Work out the finished part from the listing and answer in its coordinate system (mm). A direction names the side the tool comes from. Give positions to 0.01 mm unless a question says otherwise; leave off trailing zeros. Order: outer loops, then holes, each group sorted by start corner. A loop starts at its lowest first (then second) coordinate and runs counter-clockwise, first axis right, second up. Notation, with made-up numbers: M 25,40 L 74,40 A31 cw 74,77 Z; hole C 84,-30 d11. An arc over 180 degrees is marked long. One line per item, written item: value.
Autodesk Inventor part; units mm, degrees
ref_plane "YZ Plane" through (0, 0, 0) normal (1, 0, 0) x (0, 1, 0)
ref_plane "XZ Plane" through (0, 0, 0) normal (0, 1, 0) x (-1, 0, 0)
ref_plane "XY Plane" through (0, 0, 0) normal (0, 0, 1) x (1, 0, 0)
sketch "Sketch1" plane through (0, 0, 0) normal (0, 1, 0) x (-1, 0, 0)
  line L0 (7.8, 0) -> (7.8, -7.8)
  line L1 (7.8, -7.8) -> (-7.8, -7.8)
  line L2 (-7.8, -7.8) -> (-7.8, 7.8)
  line L3 (-7.8, 7.8) -> (7.8, 7.8)
  line L4 (7.8, 7.8) -> (7.8, 0)
  line L5 (7.8, 7.8) -> (7, 7.8)
  line L6 (-7.8, 7.8) -> (-7.8, 7.4)
  line L7 (-7.8, -7.8) -> (-7.4, -7.8)
  line L8 (7.8, -7.8) -> (7.8, -7.4)
  line L9 (0, 0) -> (7.4, 0)
  line L10 (7.4, 0) -> (7.4, -7.4)
  line L11 (7.4, -7.4) -> (-7.4, -7.4)
  line L12 (-7.4, -7.4) -> (-7.4, 7.4)
  line L13 (-7.4, 7.4) -> (7.4, 7.4)
  line L14 (7.4, 7.4) -> (7.4, 0)
  line L15 (2.7947, -7.8) -> (2.7947, -7.4)
  dimension "d1" = 7.8
  dimension "d2" = 15.6
  dimension "d3" = 15.6
  dimension "d4" = 15.6
  dimension "d5" = 7.8
  dimension "d62" = 7.4
  dimension "d63" = 7.4
  dimension "d64" = 14.8
  dimension "d65" = 14.8
  dimension "d66" = 14.8
  dimension "d68" = 0.4
extrude "Extrusion1" add sketch "Sketch1" along normal blind 18 contours L0 L1 L2 L3 L4 | L10 L11 L12 L13 L14
shell "Shell2" thickness 0.4 removed faces 2 at (2.6, 18, 0) at (2.6, 0, 0)
sketch "Sketch4" plane through (-7.8, 0, -7.8) normal (-1, 0, 0) x (0, 0, 1)
  line L0 (7.8, 0) -> (7.8, 4)
  circle A0 centre (7.8, 4) radius 0.5
  dimension "d17" = 4
  dimension "d18" = 1
hole "Hole1" at (-7.8, 4, 0) direction (1, 0, 0) diameter 1 depth 20
sketch "Sketch8" plane through (7.8, 0, 7.8) normal (1, 0, 0) x (0, 0, -1)
  line L0 (15.2, 18) -> (0.4, 18)
  line L1 (7.8, 18) -> (7.8, 14)
  circle A0 centre (7.8, 14) radius 0.5
  point P0 (7.8, 0)
  dimension "d50" = 4
  dimension "d51" = 1
hole "Hole4" at (7.8, 14, 0) direction (-1, 0, 0) diameter 1 depth 20
sketch "Sketch9" plane through (0, 0, 0) normal (0, -1, 0) x (1, 0, 0)
  line L0 (7.4, 7.4) -> (-7.4, 7.4)
  line L1 (-7.4, 7.4) -> (-7.4, 4.4)
  line L2 (-7.4, -7.4) -> (-7.4, 7.4)
  line L3 (-7.4, 4.4) -> (-7.8, 4.4)
  line L4 (-7.8, -7.8) -> (-7.8, 7.8)
  line L5 (-7.8, 4.4) -> (-7.8, 7.4)
  line L6 (-7.8, 7.4) -> (-7.4, 7.4)
  line L7 (7.4, 7.4) -> (7.4, 4.4)
  line L8 (7.4, 7.4) -> (7.4, -7.4)
  line L9 (7.4, 4.4) -> (7.8, 4.4)
  line L10 (7.8, 7.8) -> (7.8, -7.8)
  line L11 (7.8, 4.4) -> (7.8, 7.4)
  line L12 (7.8, 7.4) -> (7.4, 7.4)
  point P0 (0, 0)
  dimension "d69" = 3
  dimension "d70" = 3
extrude "Extrusion2" cut sketch "Sketch9" against normal blind 1
properties part number "Part4_cover" material "ABS Plastic"
(1) Section D-D, the plane z = 0 is taken. Give the vertices of the cut face in (x, y).
Findings:
outline: M -7.8,0 L -7.4,0 L -7.4,3.5 L -7.8,3.5 Z; M -7.8,4.5 L -7.4,4.5 L -7.4,13.5 L -7.8,13.5 Z; M -7.8,14.5 L -7.4,14.5 L -7.4,18 L -7.8,18 Z; M 7.4,0 L 7.8,0 L 7.8,3.5 L 7.4,3.5 Z; M 7.4,4.5 L 7.8,4.5 L 7.8,13.5 L 7.4,13.5 Z; M 7.4,14.5 L 7.8,14.5 L 7.8,18 L 7.4,18 Z
(2) Section A-A, the plane y = 4 is taken. Give the vertices of the cut face in (x, z), then the cut area to 3 significant figures.
Findings:
outline: M -7.8,-7.8 L 7.8,-7.8 L 7.8,-0.5 L 7.4,-0.5 L 7.4,-7.4 L -7.4,-7.4 L -7.4,-0.5 L -7.8,-0.5 Z; M -7.8,0.5 L -7.4,0.5 L -7.4,7.4 L 7.4,7.4 L 7.4,0.5 L 7.8,0.5 L 7.8,7.8 L -7.8,7.8 Z
area: 23.5 mm^2
(3) Section C-C, the plane z = -2.25 is taken. Give the vertices of the cut face in (x, y).
Findings:
outline: M -7.8,0 L -7.4,0 L -7.4,18 L -7.8,18 Z; M 7.4,0 L 7.8,0 L 7.8,18 L 7.4,18 Z
(4) Find the intervals of material crossed by probe 1 along Y at (x, z) = (-7.7, 0); probe 2 along Z at (x, y) = (-6.75, 6.25), in increasing order. Write a range as from..to.
Findings:
probe 1: y = 0..3.5, 4.5..13.5, 14.5..18
probe 2: z = -7.8..-7.4, 7.4..7.8
(5) Determine the mould class of faces 3 (the cylindrical face through (-7.603, 13.504, 0.065)), 4 (the flat face through (7.4, 9, 0)), 5 (the flat face through (-7.8, 9, 0)), 6 (the flat face through (-7.4, 9, 0)) for opening direction X: pulls with the +X half, pulls with the -X half, needs draft (parallel to the pull), parting line crosses it, or undercut.
Findings:
face 3: needs draft
face 4: undercut
face 5: pulls with the -X half
face 6: undercut
(6) Section B-B, the plane x = -1.5 is taken. Give the vertices of the cut face in (y, z).
Findings:
outline: M 0,-7.8 L 18,-7.8 L 18,-7.4 L 0,-7.4 Z; M 0,7.4 L 18,7.4 L 18,7.8 L 0,7.8 Z
(7) Which of the six approach directions +Z, -Z, +X, -X, +Y, -Y give full straight-line access (tool end or side, diameter ignored) to faces 1 (the flat face through (0, 9, 7.8)), 2 (the flat face through (0, 9, -7.4))?
Findings:
face 1: +Z, +X, -X, +Y, -Y
face 2: +Y, -Y
